```python
from build123d import *

# Parameters (mm, degrees)
SKETCH_1_R                = 70
EXTRUDE_1_DEPTH           = 60
CUT_EXTRUDE_1_DEPTH       = 116.758369028
CUT_EXTRUDE_1_DEPTH_BACK  = 116.758369028
HOLE_WIZARD_1_D           = 1.8
HOLE_WIZARD_1_CBORE_D     = 3.3
HOLE_WIZARD_1_CBORE_DEPTH = 1.8
HOLE_WIZARD_2_D           = 1.8
HOLE_WIZARD_2_CBORE_D     = 3.3
HOLE_WIZARD_2_CBORE_DEPTH = 24
SHELL_START               = 5
SHELL_1_DEPTH             = 53.180148829
SHELL_START_2             = 29
SHELL_1_2_DEPTH           = 29.180148829
SHELL_START_3             = 6.8
SHELL_1_3_DEPTH           = 22.2
FILLET_2_R                = 8


# Read off the part's stored shape, not the designer's step: 抽壳1
with BuildPart() as part:
    # 草图1 → 凸台-拉伸1 (new body)
    with BuildSketch(Plane.XY):
        Circle(SKETCH_1_R)
    extrude(amount=EXTRUDE_1_DEPTH)

    # 草图2 → 切除-拉伸1 (cut, two sides: drawn at the far end of the back side and taken through both)
    with BuildSketch(Plane(origin=(0, 0, 0), x_dir=(0, 0, -1), z_dir=(1, 0, 0)).offset(-CUT_EXTRUDE_1_DEPTH_BACK)):
        Polygon((-60, -70), (-60, 70), (-9.044167203, 70), align=None)
    extrude(amount=CUT_EXTRUDE_1_DEPTH + CUT_EXTRUDE_1_DEPTH_BACK, mode=Mode.SUBTRACT)

    # 打孔尺寸(%根据)内六角圆柱头螺钉的类型1 (through all)
    with Locations(Plane(origin=(0, 0, 0), x_dir=(-1, 0, 0), z_dir=(0, 0, -1))):
        with Locations((0, 63.75)):
            CounterBoreHole(HOLE_WIZARD_1_D / 2, HOLE_WIZARD_1_CBORE_D / 2, HOLE_WIZARD_1_CBORE_DEPTH)

    # 打孔尺寸(%根据)内六角圆柱头螺钉的类型2 (through all)
    with Locations(Plane(origin=(0, 0, 0), x_dir=(-1, 0, 0), z_dir=(0, 0, -1))):
        with Locations((-63.75, 0), (63.75, 0)):
            CounterBoreHole(HOLE_WIZARD_2_D / 2, HOLE_WIZARD_2_CBORE_D / 2, HOLE_WIZARD_2_CBORE_DEPTH)

    # 抽壳1 outline → 抽壳1 (cut)
    with BuildSketch(Plane.XY.offset(SHELL_START)):
        with BuildLine():
            ThreePointArc((-64.665411765, -6.586692744), (0, -65), (64.665411765, -6.586692744))
            ThreePointArc((64.665411765, -6.586692744), (57.1, 0), (64.665411765, 6.586692744))
            ThreePointArc((64.665411765, 6.586692744), (45.961940777, 45.961940777), (6.586692744, 64.665411765))
            ThreePointArc((6.586692744, 64.665411765), (0, 57.1), (-6.586692744, 64.665411765))
            ThreePointArc((-6.586692744, 64.665411765), (-45.961940777, 45.961940777), (-64.665411765, 6.586692744))
            ThreePointArc((-64.665411765, 6.586692744), (-57.1, 0), (-64.665411765, -6.586692744))
        make_face()
    extrude(amount=SHELL_1_DEPTH, mode=Mode.SUBTRACT)

    # Shell 1 2 outline → Shell 1 2 (cut)
    with BuildSketch(Plane.XY.offset(SHELL_START_2)):
        with BuildLine():
            ThreePointArc((64.665411765, -6.586692744), (64.703469597, -6.2016951), (64.739235294, -5.81647776))
            ThreePointArc((64.739235294, -5.81647776), (57.85, 0), (64.739235294, 5.81647776))
            ThreePointArc((64.739235294, 5.81647776), (64.703469597, 6.2016951), (64.665411765, 6.586692744))
            ThreePointArc((64.665411765, 6.586692744), (57.1, 0), (64.665411765, -6.586692744))
        make_face()
        with BuildLine():
            ThreePointArc((-64.739235294, -5.81647776), (-64.703469597, -6.2016951), (-64.665411765, -6.586692744))
            ThreePointArc((-64.665411765, -6.586692744), (-57.1, 0), (-64.665411765, 6.586692744))
            ThreePointArc((-64.665411765, 6.586692744), (-64.703469597, 6.2016951), (-64.739235294, 5.81647776))
            ThreePointArc((-64.739235294, 5.81647776), (-57.85, 0), (-64.739235294, -5.81647776))
        make_face()
    extrude(amount=SHELL_1_2_DEPTH, mode=Mode.SUBTRACT)

    # Shell 1 3 outline → Shell 1 3 (cut)
    with BuildSketch(Plane.XY.offset(SHELL_START_3)):
        with BuildLine():
            ThreePointArc((-6.586692744, 64.665411765), (0, 57.1), (6.586692744, 64.665411765))
            ThreePointArc((6.586692744, 64.665411765), (6.2016951, 64.703469597), (5.81647776, 64.739235294))
            ThreePointArc((5.81647776, 64.739235294), (0, 57.85), (-5.81647776, 64.739235294))
            ThreePointArc((-5.81647776, 64.739235294), (-6.2016951, 64.703469597), (-6.586692744, 64.665411765))
        make_face()
    extrude(amount=SHELL_1_3_DEPTH, mode=Mode.SUBTRACT)

    # 圆角2
    # the kernel refuses this fillet: 8 mm, written as the material it takes off along each edge
    with BuildSketch(Plane(origin=(0, 0, 0), x_dir=(1, 0, 0), z_dir=(0, -1, 0))) as fillet_2_piece_1:
        with BuildLine():
            CenterArc((70 - FILLET_2_R, FILLET_2_R), FILLET_2_R, 270, 90)
            Line((70 - FILLET_2_R, 0), (70, 0))
            Line((70, 0), (70, FILLET_2_R))
        make_face()
    revolve(axis=Axis((0, 0, 0), (0, 0, 1)), mode=Mode.SUBTRACT)


solid = part.part
```
Verification items for the finished model (mm, model axes). A direction names the side the tool comes from. Coordinates: 2 decimals unless noted, no trailing zeros. Loops run counter-clockwise (first coordinate to the right, second up) from the corner with the lowest first, then second, coordinate; pieces in that order, holes last. Notation, with made-up numbers: (78, 72.5) -> (88, 72.5) arc R17 cw to (88, 88.5) -> close; hole circle Ø1 at (8, 81.25). An arc over 180 degrees is marked (long way). Put each result on its own line as item: value.
1. Gauge pin test, flat ends, axial feed: P1, Ø8, axis at x = 19, z = 28, coming from the -Y side; P2, Ø3, axis at x = 0, y = 63.75, coming from the -Z side; P3, Ø1.5, axis at x = 6, z = 44, coming from the +Y side. Record the tip position at first contact, or that the pin passes through.
Result set:
P1: stops at y = -68.37
P2: stops at z = 1.8
P3: stops at y = -64.65
2. Section check A-A, the plane z = 21. Record the boundary of the cut face in (x, y), then the cut area to 3 significant figures.
Result set:
outline: (-64.67, -6.59) arc R6.65 ccw (long way) to (-64.67, 6.59) arc R65 cw to (-53.34, 37.15) -> (-59.33, 37.15) arc R70 ccw (long way) to (59.33, 37.15) -> (53.34, 37.15) arc R65 cw to (64.67, 6.59) arc R6.65 ccw (long way) to (64.67, -6.59) arc R65 cw to start; hole circle Ø3.3 at (-63.75, 0); hole circle Ø3.3 at (63.75, 0)
area: 1,610 mm^2
3. Mould release check, pull along X, two halves, no side actions. Record for faces 4 (the face through (61.9, 0.33, 34.4)), 5 (the face through (57.1, -0.16, 16.83)), 6 (the face through (-15.175, -68.335, 27.858)): pulls with the +X half, pulls with the -X half, needs draft (parallel to the pull), parting line crosses it, or undercut.
Result set:
face 4: needs draft
face 5: undercut
face 6: parting line crosses it
4. Thickness scan on line 1 (X direction, y = 0, z = 32); line 2 (X direction, y = 0, z = 28.25); line 3 (Y direction, x = 0, z = 7.5). Record the ranges inside material, lowest first.
Result set:
line 1: x = -70 to -64.65, -62.85 to -57.85, 57.85 to 62.85, 64.65 to 70
line 2: x = -70 to -64.65, -62.85 to -57.1, 57.1 to 62.85, 64.65 to 70
line 3: y = -69.98 to -65, 57.85 to 62.85, 64.65 to 69.98
5. Tool access check on faces 1 (the face through (-1, 63, 1.8)), 2 (the face through (-1, 1, 0)), 3 (the face through (-1, 1, 5)). Record the directions out of +Z, -Z, +X, -X, +Y, -Y that give a thin tool (end or side, any length) a straight path to the whole face; none if there is none.
Result set:
face 1: -Z
face 2: -Z, +X, -X, +Y, -Y
face 3: +Z
6. Section check B-B, the plane z = 48. Record the boundary of the cut face in (x, y).
Result set:
outline: (-59.4, -37.03) arc R70 ccw to (59.4, -37.03) -> (53.42, -37.03) arc R65 cw to (-53.42, -37.03) -> close
